Autodesk Inventor part; units mm, degrees
ref_plane "YZ Plane" through (0, 0, 0) normal (1, 0, 0) x (0, 1, 0)
ref_plane "XZ Plane" through (0, 0, 0) normal (0, 1, 0) x (-1, 0, 0)
ref_plane "XY Plane" through (0, 0, 0) normal (0, 0, 1) x (1, 0, 0)
sketch "Sketch1" plane through (0, 0, 0) normal (0, 1, 0) x (-1, 0, 0)
  line L0 (0, 0) -> (30, 0)
  line L1 (30, 0) -> (30, -96)
  line L2 (30, -96) -> (0, -96)
  line L3 (0, -96) -> (0, 0)
  dimension "d0" = 30
  dimension "d1" = 96
extrude "Extrusion1" add sketch "Sketch1" along normal blind 13
sketch "Sketch2" plane through (0, 13, 0) normal (0, 1, 0) x (1, 0, 0)
  line L0 (-30, 96) -> (-30, 0)
  line L1 (0, 0) -> (0, 96)
  line L2 (-30, 0) -> (0, 0)
  line L3 (0, 0) -> (0, 5.5)
  line L4 (0, 5.5) -> (-30, 5.5)
  line L5 (-30, 5.5) -> (-30, 0)
  line L6 (0, 96) -> (-30, 96)
  line L7 (-30, 96) -> (-30, 90.5)
  line L8 (-30, 90.5) -> (0, 90.5)
  line L9 (0, 90.5) -> (0, 96)
  line L10 (-30, 96) -> (0, 96)
  line L11 (0, 96) -> (0, 90.5)
  line L12 (0, 90.5) -> (-30, 90.5)
  line L13 (-30, 90.5) -> (-30, 96)
  dimension "d4" = 5.5
  dimension "d5" = 5.5
extrude "Extrusion2" add sketch "Sketch2" along normal blind 15.5 contours L4 L1 L2 L0
sketch "Sketch4" plane through (0, 13, 0) normal (0, 1, 0) x (1, 0, 0)
  line L0 (0, 0) -> (0, 96)
  line L1 (-30, 96) -> (-30, 0)
  line L2 (0, 96) -> (-30, 96)
  line L3 (-30, 96) -> (-30, 90.5)
  line L4 (-30, 90.5) -> (0, 90.5)
  line L5 (0, 90.5) -> (0, 96)
  point P0 (0, 90.5)
  dimension "d8" = 5.5
extrude "Extrusion3" add sketch "Sketch4" along normal blind 22
sketch "Sketch6" plane through (0, 0, -96) normal (0, 0, -1) x (-1, 0, 0)
  line L0 (30, 35) -> (0, 35) construction
  line L1 (30, 0) -> (30, 28.5)
  line L2 (0, 35) -> (30, 35) construction
  line L3 (30, 35) -> (30, 7) construction
  line L4 (30, 7) -> (0, 7) construction
  line L5 (0, 7) -> (0, 35) construction
  line L6 (0, 7) -> (30, 35) construction
  line L7 (0, 35) -> (30, 7) construction
  circle A0 centre (15, 21) radius 3
  point P0 (0, 0)
  dimension "d11" = 28
  dimension "d12" = 6
extrude "Extrusion4" add sketch "Sketch6" against normal up to surface (90.5 mm away)
sketch "Sketch7" plane through (0, 0, -96) normal (0, 0, -1) x (-1, 0, 0)
  line L0 (30, 0) -> (30, 28.5)
  line L1 (30, 35) -> (0, 35)
  line L2 (1, 35) -> (29, 35)
  line L3 (29, 35) -> (29, 7)
  line L4 (29, 7) -> (1, 7)
  line L5 (1, 7) -> (1, 35)
  point P0 (0, 0)
  point P1 (15, 35)
  dimension "d15" = 28
extrude "Extrusion5" add sketch "Sketch7" along normal blind 30
sketch "Sketch8" plane through (0, 0, 0) normal (0, -1, 0) x (1, 0, 0)
  circle A0 centre (-6.5, -75.5) radius 1.7
  circle A1 centre (-23.5, -75.5) radius 1.7
  circle A2 centre (-6.5, -20.5) radius 1.7
  circle A3 centre (-23.5, -20.5) radius 1.7
  line L0 (0, 0) -> (0, -96)
  line L1 (-30, 0) -> (0, 0)
  line L2 (-30, -96) -> (-30, 0)
  line L3 (0, -96) -> (-30, -96)
  dimension "d18" = 3.4
  dimension "d19" = 55
  dimension "d20" = 6.5
  dimension "d21" = 20.5
  dimension "d22" = 6.5
  dimension "d25" = 17
  dimension "d26" = 20.5
extrude "Extrusion6" cut sketch "Sketch8" against normal blind 30 contours A0 | A1 | A2 | A3
equation "\"d5\" = d4"
equation "\"d22\" = d20"
properties part number "AE_50MM_STAGE"
Check sheet for the modelled part. Datum: model origin and axes. Units: mm. A direction names the side the tool comes from. Round coordinates to 2 decimals unless told otherwise and drop trailing zeros. Order: outer loops, then holes, each group sorted by start corner. A loop starts at its lowest first (then second) coordinate and runs counter-clockwise, first axis right, second up. Notation, with made-up numbers: M 54.25,-23.5 L 96.25,-23.5 A18 cw 96.25,9.5 Z; hole C -34.75,-4.75 d8. An arc over 180 degrees is marked long. One line per item, written item: value. Start each with the question number.
1. Section check B-B on z = -20.5. Enter the section's corners in (x, y), and give its area (3 significant figures).
2. Section check D-D on y = 33.5. Enter the section's corners in (x, z).
3. Gauge pin test, flat ends, axial feed: P1, Ø8.5, axis at y = 26.5, z = -117.5, coming from the +X side; P2, Ø4, axis at x = -6.5, z = -20.5, coming from the +Y side; P3, Ø1.6, axis at x = -10.5, z = -2, coming from the +Y side. Record the tip position at first contact, or that the pin passes through.
4. Release check for a two-part mould opening along Z. For faces 1 (the flat face through (-15, 7, -111)), 2 (the cylindrical face through (-12.6, 19.2, -48.6)), 3 (the cylindrical face through (-6.721, 6.409, -18.814)), 4 (the flat face through (-15, 14, 0)) record: released by +Z, released by -Z, zero draft, split by the parting line, or undercut.
5. Section check C-C on y = 4.5. Enter the section's corners in (x, z), and give its area (3 significant figures).
6. Access from +Z, -Z, +X, -X, +Y, -Y to the whole of each face (thin tool, end or side, straight path). Record for faces 5 (the flat face through (-15, 21, -126)), 6 (the flat face through (-15, 28.5, -3)), 7 (the flat face through (-29, 21, -111)), 8 (the cylindrical face through (-22.7, 6.4, -77)), 9 (the flat face through (-1, 21, -111)).
7. Scan lines: line 1 along Z through (x, y) = (-23.25, 7.5); line 2 along X through (y, z) = (2.5, -75.5); line 3 along Z through (x, y) = (-23.5, 4). Record each from-to range of solid material in increasing order.
8. Section check A-A on x = -6.5. Enter the section's corners in (y, z).
Results found:
1. outline: M -30,0 L -25.2,0 L -25.2,13 L -30,13 Z; M -21.8,0 L -8.2,0 L -8.2,13 L -21.8,13 Z; C -15,21 d6; M -4.8,0 L 0,0 L 0,13 L -4.8,13 Z
1. area: 330 mm^2
2. outline: M -30,-96 L -29,-96 L -29,-126 L -1,-126 L -1,-96 L 0,-96 L 0,-90.5 L -30,-90.5 Z
3. P1: x = -1
3. P2: y = 13
3. P3: y = 28.5
4. face 1: zero draft
4. face 2: undercut
4. face 3: undercut
4. face 4: released by +Z
5. outline: M -30,-96 L 0,-96 L 0,0 L -30,0 Z; hole C -23.5,-75.5 d3.4; hole C -23.5,-20.5 d3.4; hole C -6.5,-75.5 d3.4; hole C -6.5,-20.5 d3.4
5. area: 2,840 mm^2
6. face 5: -Z, +X, -X, +Y, -Y
6. face 6: +Z, +X, -X, +Y
6. face 7: -Z, -X, +Y, -Y
6. face 8: +Y, -Y
6. face 9: -Z, +X, +Y, -Y
7. line 1: -126 to -77.18, -73.82 to -22.18, -18.82 to 0
7. line 2: -30 to -25.2, -21.8 to -8.2, -4.8 to 0
7. line 3: -96 to -77.2, -73.8 to -22.2, -18.8 to 0
8. outline: M 0,-96 L 7,-96 L 7,-126 L 35,-126 L 35,-90.5 L 13,-90.5 L 13,-77.2 L 0,-77.2 Z; M 0,-73.8 L 13,-73.8 L 13,-22.2 L 0,-22.2 Z; M 0,-18.8 L 13,-18.8 L 13,-5.5 L 28.5,-5.5 L 28.5,0 L 0,0 Z
